For this review, use the dimensioned drawing (mm, ordinates from the lowest corner) and the shaded views. Give positions to 0.01 mm unless a question says otherwise; leave off trailing zeros. Loops run counter-clockwise (first coordinate to the right, second up) from the corner with the lowest first, then second, coordinate; pieces in that order, holes last. Notation, with made-up numbers: M -25,67 L 5,67 A12 ccw 5,82 Z; hole C 82.25,-32 d3. An arc over 180 degrees is marked long. Use a Markdown table: item, result. Add a question column.
(1) For probe 1 along X at (y, z) = (25, 13); probe 2 along Y at (x, z) = (12.5, 9.5); probe 3 along X at (y, z) = (19.5, 15.25), list the stretches that pass through material, from the lowest coordinate up.
(2) Add section A-A, the plane z = 17.75. Give the boundary of the cut face in (x, y).
(3) Draft analysis for pull direction Y (two halves, no side actions). For the marked faces 1, 2, 3 and 4, state which applies: pulls with the +Y half, pulls with the -Y half, needs draft (parallel to the pull), parting line crosses it, or undercut.
(4) Add section B-B, the plane x = 57.5. Give the boundary of the cut face in (y, z), then the cut area to 3 significant figures.
(5) Add section C-C, the plane y = 25. Give the boundary of the cut face in (x, z), then the cut area to 3 significant figures.
(6) Insertion check: pin 1 Ø12 at (x, y) = (51.5, 22.5) entering from -Z; pin 2 Ø11 at (x, y) = (12.5, 25) entering from -Z. Each pin has a flat end and moves straight along its axis. Give the tip position at first contact, or say it passes through.
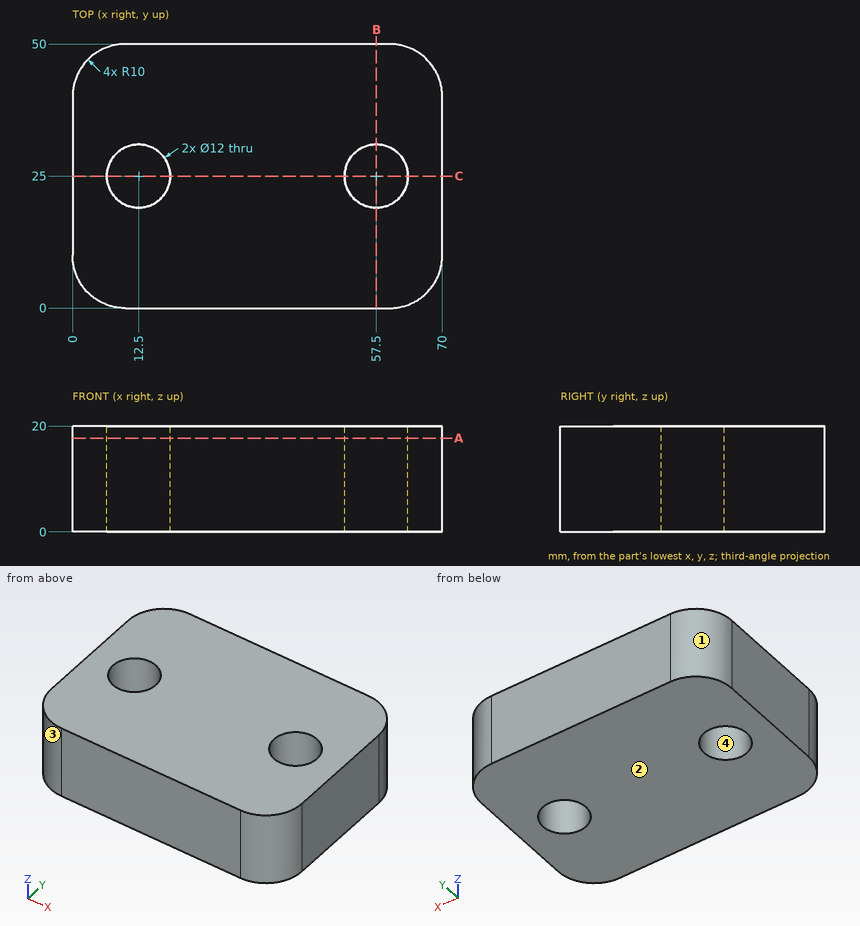
Established:
| question | item | result |
|---|---|---|
| 1 | probe 1 | 0 to 6.5, 18.5 to 51.5, 63.5 to 70 |
| 1 | probe 2 | 0 to 19, 31 to 50 |
| 1 | probe 3 | 0 to 10.1, 14.9 to 55.1, 59.9 to 70 |
| 2 | outline | M 0,10 A10 ccw 10,0 L 60,0 A10 ccw 70,10 L 70,40 A10 ccw 60,50 L 10,50 A10 ccw 0,40 Z; hole C 12.5,25 d12; hole C 57.5,25 d12 |
| 3 | face 1 | pulls with the +Y half |
| 3 | face 2 | needs draft |
| 3 | face 3 | pulls with the -Y half |
| 3 | face 4 | undercut |
| 4 | outline | M 0,0 L 19,0 L 19,20 L 0,20 Z; M 31,0 L 50,0 L 50,20 L 31,20 Z |
| 4 | area | 760 mm^2 |
| 5 | outline | M 0,0 L 6.5,0 L 6.5,20 L 0,20 Z; M 18.5,0 L 51.5,0 L 51.5,20 L 18.5,20 Z; M 63.5,0 L 70,0 L 70,20 L 63.5,20 Z |
| 5 | area | 920 mm^2 |
| 6 | pin 1 | z = 0 |
| 6 | pin 2 | through |
